```python
from build123d import *

# Parameters (mm, degrees)
SKETCH1_W           = 94.2086
SKETCH1_H           = 101
BOSS_EXTRUDE1_DEPTH = 26.1
SKETCH2_R           = 5.461
BOSS_EXTRUDE2_DEPTH = 2.54
SKETCH3_W           = 80.593596518
SKETCH3_H           = 16.42098599
CUT_EXTRUDE1_DEPTH  = 5


with BuildPart() as part:
    # Sketch1 → Boss-Extrude1 (new body)
    with BuildSketch(Plane(origin=(0, 0, 0), x_dir=(1, 0, 0), z_dir=(0, 1, 0))):
        with Locations((47.1043, 50.5)):
            Rectangle(SKETCH1_W, SKETCH1_H)
        with BuildLine():
            ThreePointArc((22, 56.0118), (23.9685, 57.9803), (25.937, 56.0118))
            Line((25.937, 56.0118), (25.937, 53.182647668))
            ThreePointArc((25.937, 53.182647668), (26.321327104, 52.852827104), (26.651147668, 52.4685))
            Line((26.651147668, 52.4685), (29.8232, 52.4685))
            ThreePointArc((29.8232, 52.4685), (31.7917, 50.5), (29.8232, 48.5315))
            Line((29.8232, 48.5315), (26.651147668, 48.5315))
            ThreePointArc((26.651147668, 48.5315), (26.321327104, 48.147172896), (25.937, 47.817352332))
            Line((25.937, 47.817352332), (25.937, 44.9882))
            ThreePointArc((25.937, 44.9882), (23.9685, 43.0197), (22, 44.9882))
            Line((22, 44.9882), (22, 47.817352332))
            ThreePointArc((22, 47.817352332), (20.6411, 50.5), (22, 53.182647668))
            Line((22, 53.182647668), (22, 56.0118))
        make_face(mode=Mode.SUBTRACT)
        with BuildLine():
            ThreePointArc((68.2716, 56.0118), (70.2401, 57.9803), (72.2086, 56.0118))
            Line((72.2086, 56.0118), (72.2086, 53.182647668))
            ThreePointArc((72.2086, 53.182647668), (72.592927104, 52.852827104), (72.922747668, 52.4685))
            Line((72.922747668, 52.4685), (76.0948, 52.4685))
            ThreePointArc((76.0948, 52.4685), (78.0633, 50.5), (76.0948, 48.5315))
            Line((76.0948, 48.5315), (72.922747668, 48.5315))
            ThreePointArc((72.922747668, 48.5315), (72.592927104, 48.147172896), (72.2086, 47.817352332))
            Line((72.2086, 47.817352332), (72.2086, 44.9882))
            ThreePointArc((72.2086, 44.9882), (70.2401, 43.0197), (68.2716, 44.9882))
            Line((68.2716, 44.9882), (68.2716, 47.817352332))
            ThreePointArc((68.2716, 47.817352332), (66.9127, 50.5), (68.2716, 53.182647668))
            Line((68.2716, 53.182647668), (68.2716, 56.0118))
        make_face(mode=Mode.SUBTRACT)
    extrude(amount=BOSS_EXTRUDE1_DEPTH)

    # Sketch2 → Boss-Extrude2 (add)
    with BuildSketch(Plane.XZ):
        with Locations(Location((11.938, -20.32, 0), (0, 0, 90))):
            Circle(SKETCH2_R)
        with Locations(Location((82.2706, -20.32, 0), (0, 0, 90))):
            Circle(SKETCH2_R)
        with Locations(Location((11.938, -85.76, 0), (0, 0, 90))):
            Circle(SKETCH2_R)
        with Locations(Location((82.2706, -85.76, 0), (0, 0, 90))):
            Circle(SKETCH2_R)
    extrude(amount=BOSS_EXTRUDE2_DEPTH)

    # Sketch3 → Cut-Extrude1 (cut)
    with BuildSketch(Plane(origin=(0, 0, -101), x_dir=(-1, 0, 0), z_dir=(0, 0, -1))):
        with Locations((-47.1043, 13.05)):
            Rectangle(SKETCH3_W, SKETCH3_H)
    extrude(amount=-CUT_EXTRUDE1_DEPTH, mode=Mode.SUBTRACT)


solid = part.part
```
Read the model definition and answer for the solid it produces. Units are mm, in the model's axes. A direction names the side the tool comes from. Round coordinates to 2 decimals unless told otherwise and drop trailing zeros. Write each loop counter-clockwise with the first axis right and the second up, starting at its lowest first coordinate (ties: lowest second). Pieces come first, ordered by that corner, then holes. Notation, with made-up numbers: (70, -15) -> (89, -15) arc R33 ccw to (89, 20) -> close; hole circle Ø11 at (48.25, 35). An arc over 180 degrees is marked (long way). Answer in a Markdown table with one row per item. Add a question column.
1) Determine the mould class of faces 5 (the face through (94.209, 13, -50)), 6 (the face through (48, 13, -96)), 7 (the face through (82, -2.54, -86)) for opening direction X: pulls with the +X half, pulls with the -X half, needs draft (parallel to the pull), parting line crosses it, or undercut.
2) Given P1, Ø1.5, axis at x = 23.5, z = -24, coming from the -Y side; P2, Ø2.5, axis at x = 75, y = 9, coming from the -Z side, each flat-ended and moving along its own axis, determine where each tip first touches the part or whether it passes through.
3) Consider line 1 (Z direction, x = 66.5, y = 10.5); line 2 (Y direction, x = 22, z = -23); line 3 (X direction, y = 20.5, z = -51). Determine where each line is inside the solid, lowest interval first.
4) Find section D-D, the plane z = -34.5. Determine the outline of the cut face in (x, y).
5) Find section B-B, the plane z = -50.5. Determine the outline of the cut face in (x, y).
6) Find section A-A, the plane y = 19. State how many separate pieces and enclosed holes the cut face has, and give its area (3 significant figures).
7) Which of the six approach directions +Z, -Z, +X, -X, +Y, -Y give full straight-line access (tool end or side, diameter ignored) to faces 1 (the face through (6.808, 13, -99)), 2 (the face through (25.937, 13, -55)), 3 (the face through (15.261, -1.252, -24.654)), 4 (the face through (0, 13, -50))?
8) Find section C-C, the plane z = -85.76. Determine the outline of the cut face in (x, y).
Findings below:
| question | item | result |
|---|---|---|
| 1 | face 5 | pulls with the +X half |
| 1 | face 6 | undercut |
| 1 | face 7 | needs draft |
| 2 | P1 | y = 0 |
| 2 | P2 | z = -96 |
| 3 | line 1 | -96 to 0 |
| 3 | line 2 | 0 to 26.1 |
| 3 | line 3 | 0 to 20.68, 31.73 to 66.95, 78 to 94.21 |
| 4 | outline | (0, 0) -> (94.21, 0) -> (94.21, 26.1) -> (0, 26.1) -> close |
| 5 | outline | (0, 0) -> (20.64, 0) -> (20.64, 26.1) -> (0, 26.1) -> close; (31.79, 0) -> (66.91, 0) -> (66.91, 26.1) -> (31.79, 26.1) -> close; (78.06, 0) -> (94.21, 0) -> (94.21, 26.1) -> (78.06, 26.1) -> close |
| 6 | separate pieces | 1 |
| 6 | enclosed holes | 2 |
| 6 | area | 8,950 mm² |
| 7 | face 1 | -Z |
| 7 | face 2 | +Y, -Y |
| 7 | face 3 | -Y |
| 7 | face 4 | +Z, -Z, -X, +Y, -Y |
| 8 | outline | (0, 0) -> (6.48, 0) -> (6.48, -2.54) -> (17.4, -2.54) -> (17.4, 0) -> (76.81, 0) -> (76.81, -2.54) -> (87.73, -2.54) -> (87.73, 0) -> (94.21, 0) -> (94.21, 26.1) -> (0, 26.1) -> close |
